```python
from build123d import *

# Parameters (mm, degrees)
PLATES_BASE_OUTLINE_W   = 90
PLATES_BASE_OUTLINE_H   = 60
PLATES_BASE_OUTLINE_R   = 1.5
PLATES_BASE_OUTLINE_W_2 = 76
PLATES_BASE_OUTLINE_H_2 = 20
PLATES_BASE_DEPTH       = 1.6
SKETCH_4_W              = 78
SKETCH_4_H              = 48
CUT_EXTRUDE_1_DEPTH     = 94.689835584
SKETCH_7_W              = 6
SKETCH_7_H              = 6
EXTRUDE_4_DEPTH         = 1.6
SKETCH_8_W              = 6
SKETCH_8_H              = 48
EXTRUDE_5_DEPTH         = 1.6
SKETCH_10_R             = 1.5
CUT_EXTRUDE_4_DEPTH     = 1.6


# Read off the part's stored shape, not the designer's step: plates=base
with BuildPart() as part:
    # plates=base outline → plates=base (new body)
    with BuildSketch(Plane.XY):
        with Locations((-41.587399894, 5.746992481)):
            Rectangle(PLATES_BASE_OUTLINE_W, PLATES_BASE_OUTLINE_H)
        with Locations((-83.587399894, -21.253007519)):
            Circle(PLATES_BASE_OUTLINE_R, mode=Mode.SUBTRACT)
        with Locations((0.412600106, -21.253007519)):
            Circle(PLATES_BASE_OUTLINE_R, mode=Mode.SUBTRACT)
        with Locations((-41.587399894, -7.253007519)):
            Rectangle(PLATES_BASE_OUTLINE_W_2, PLATES_BASE_OUTLINE_H_2, mode=Mode.SUBTRACT)
        with Locations((-78.587399894, 5.746992481)):
            Circle(PLATES_BASE_OUTLINE_R, mode=Mode.SUBTRACT)
        with Locations((-83.587399894, 32.746992481)):
            Circle(PLATES_BASE_OUTLINE_R, mode=Mode.SUBTRACT)
        with Locations((-41.587399894, 18.746992481)):
            Rectangle(PLATES_BASE_OUTLINE_W_2, PLATES_BASE_OUTLINE_H_2, mode=Mode.SUBTRACT)
        with Locations((-4.587399894, 5.746992481)):
            Circle(PLATES_BASE_OUTLINE_R, mode=Mode.SUBTRACT)
        with Locations((0.412600106, 32.746992481)):
            Circle(PLATES_BASE_OUTLINE_R, mode=Mode.SUBTRACT)
    extrude(amount=PLATES_BASE_DEPTH)

    # ｽｹｯﾁ4 → ｶｯﾄ - 押し出し1 (cut, through all)
    with BuildSketch(Plane.XY.offset(1.6)):
        with Locations((-41.587399894, 5.746992481)):
            Rectangle(SKETCH_4_W, SKETCH_4_H)
    extrude(amount=-CUT_EXTRUDE_1_DEPTH, mode=Mode.SUBTRACT)

    # ｽｹｯﾁ7 → ﾎﾞｽ - 押し出し4 (add)
    with BuildSketch(Plane.XY.offset(1.6)):
        with Locations((0.412600106, -27.253007519)):
            Rectangle(SKETCH_7_W, SKETCH_7_H)
        with Locations((-57.587399894, -27.253007519)):
            Rectangle(SKETCH_7_W, SKETCH_7_H)
    extrude(amount=-EXTRUDE_4_DEPTH)

    # ｽｹｯﾁ8 → ﾎﾞｽ - 押し出し5 (add)
    with BuildSketch(Plane.XY.offset(1.6)):
        with Locations((-57.587399894, 5.746992481)):
            Rectangle(SKETCH_8_W, SKETCH_8_H)
    extrude(amount=-EXTRUDE_5_DEPTH)

    # ｽｹｯﾁ10 → ｶｯﾄ - 押し出し4 (cut)
    with BuildSketch(Plane.XY.offset(1.6)):
        with Locations((0.412600106, -27.253007519)):
            Circle(SKETCH_10_R)
        with Locations((-57.587399894, -27.253007519)):
            Circle(SKETCH_10_R)
        with Locations((-57.587399894, 21.746992481)):
            Circle(SKETCH_10_R)
        with Locations((0.412600106, 21.746992481)):
            Circle(SKETCH_10_R)
    extrude(amount=-CUT_EXTRUDE_4_DEPTH, mode=Mode.SUBTRACT)


solid = part.part
```
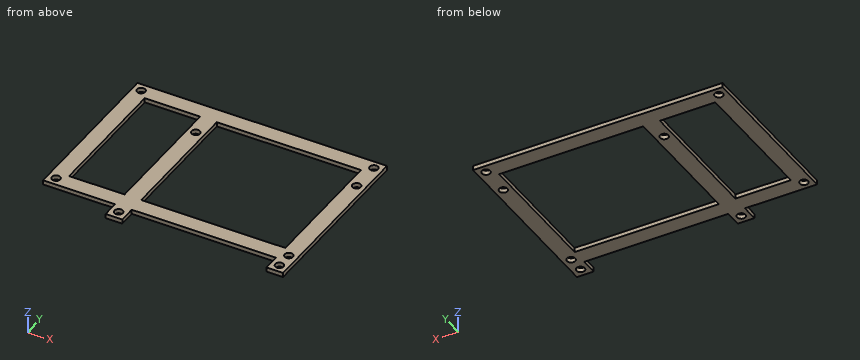
Build history of the part. All positions in model axes, mm. Give positions to 0.01 mm unless a question says otherwise; leave off trailing zeros. Loops run counter-clockwise (first coordinate to the right, second up) from the corner with the lowest first, then second, coordinate; pieces in that order, holes last.
1) Band-saw the part on C-C on z = 0.95. State how many separate pieces and enclosed holes the cut face has, then the cut area to 3 significant figures.
Values follow:
separate pieces: 1
enclosed holes: 10
area: 1,960 mm2
2) Probe line 1 along X through (y, z) = (17, 1.1); line 2 along Y through (x, z) = (-15.5, 1.3); line 3 along X through (y, z) = (20.5, 1.2). List the from-to ranges inside material, lowest first.
Values follow:
line 1: x = -86.59 to -80.59, -60.59 to -54.59, -2.59 to 3.41
line 2: y = -24.25 to -18.25, 29.75 to 35.75
line 3: x = -86.59 to -80.59, -60.59 to -58.42, -56.75 to -54.59, -2.59 to -0.42, 1.25 to 3.41
3) Band-saw the part on B-B on y = -13.5. List the corners of the cut face in (x, z).
Values follow:
outline: (-86.59, 0) - (-80.59, 0) - (-80.59, 1.6) - (-86.59, 1.6) - close; (-60.59, 0) - (-54.59, 0) - (-54.59, 1.6) - (-60.59, 1.6) - close; (-2.59, 0) - (3.41, 0) - (3.41, 1.6) - (-2.59, 1.6) - close
4) Drop a flat-ended pin along its axis: P1, Ø0.8, axis at x = -31, z = 1, coming from the -Y side. Give the stop position or say it passes through.
Values follow:
P1: stops at y = -24.25
5) Band-saw the part on A-A on x = -67. List the corners of the cut face in (y, z).
Values follow:
outline: (-24.25, 0) - (-18.25, 0) - (-18.25, 1.6) - (-24.25, 1.6) - close; (29.75, 0) - (35.75, 0) - (35.75, 1.6) - (29.75, 1.6) - close
